Here's the drawing with two shaded views (mm, measured from the low corner). I have some questions. A direction names the side the tool comes from. Coordinates: 2 decimals unless noted, no trailing zeros. Loops run counter-clockwise (first coordinate to the right, second up) from the corner with the lowest first, then second, coordinate; pieces in that order, holes last.
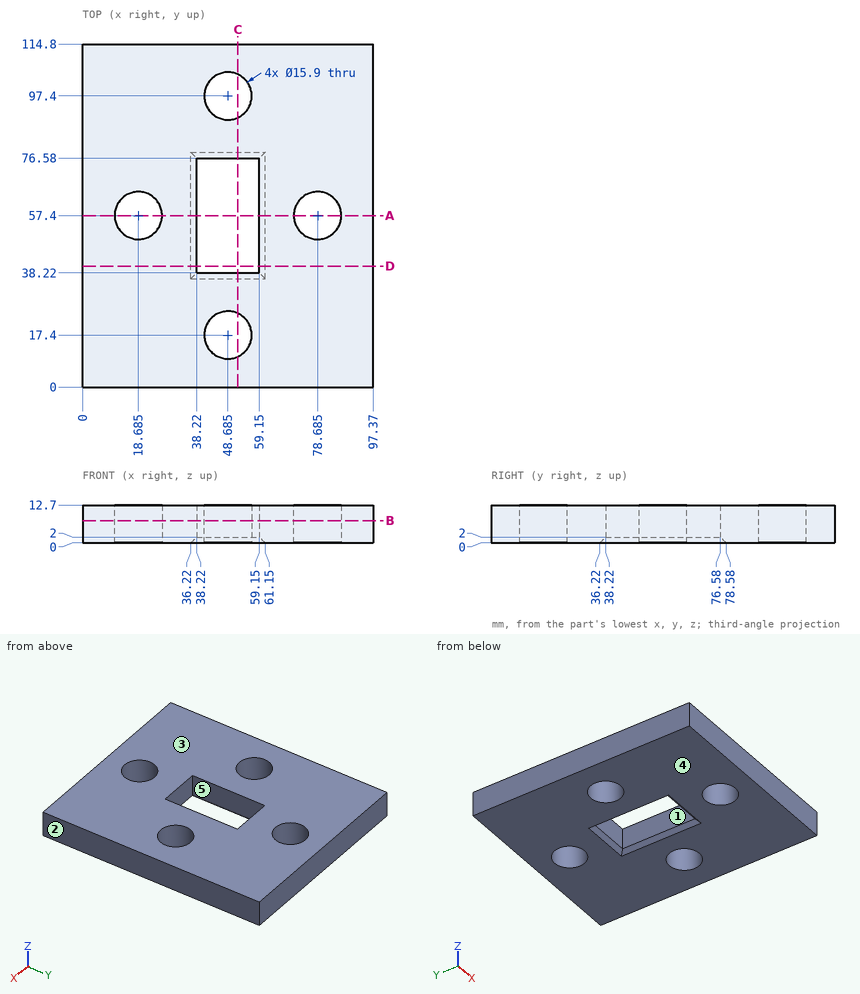
(1) I want a section at B-B on z = 7.5. Write out the boundary of the cut face in (x, y) (3 decimals), then the cut area to 3 significant figures.
Check values:
outline: (0, 0) - (97.37, 0) - (97.37, 114.8) - (0, 114.8) - close; hole circle Ø15.9 at (18.685, 57.4); hole (38.22, 38.22) - (59.15, 38.22) - (59.15, 76.58) - (38.22, 76.58) - close; hole circle Ø15.9 at (48.685, 17.4); hole circle Ø15.9 at (48.685, 97.4); hole circle Ø15.9 at (78.685, 57.4)
area: 9,580 mm2
(2) I want a section at A-A on y = 57.4. Write out the boundary of the cut face in (x, z) (3 decimals).
Check values:
outline: (0, 0) - (10.735, 0) - (10.735, 12.7) - (0, 12.7) - close; (26.635, 0) - (36.22, 0) - (38.22, 2) - (38.22, 12.7) - (26.635, 12.7) - close; (59.15, 2) - (61.15, 0) - (70.735, 0) - (70.735, 12.7) - (59.15, 12.7) - close; (86.635, 0) - (97.37, 0) - (97.37, 12.7) - (86.635, 12.7) - close
(3) I want a section at D-D on y = 40.5. Write out the boundary of the cut face in (x, z), then the cut area to 3 significant figures.
Check values:
outline: (0, 0) - (36.22, 0) - (38.22, 2) - (38.22, 12.7) - (0, 12.7) - close; (59.15, 2) - (61.15, 0) - (97.37, 0) - (97.37, 12.7) - (59.15, 12.7) - close
area: 967 mm2
(4) I want a section at C-C on x = 52. Write out the boundary of the cut face in (y, z).
Check values:
outline: (0, 0) - (10.17, 0) - (10.17, 12.7) - (0, 12.7) - close; (24.63, 0) - (36.22, 0) - (38.22, 2) - (38.22, 12.7) - (24.63, 12.7) - close; (76.58, 2) - (78.58, 0) - (90.17, 0) - (90.17, 12.7) - (76.58, 12.7) - close; (104.63, 0) - (114.8, 0) - (114.8, 12.7) - (104.63, 12.7) - close
(5) I'm going to push a flat-ended pin straight in: pin 1 (9.5 mm diameter, centred on x = 48.685, y = 97.4, fed in from -Z). Where does the tip first touch, or does it pass through?
Check values:
pin 1: passes through
(6) If we mould it in two halves opening along X, with no side actions, what happens to the marked faces 1, 2 and 3? For each: released by +X, released by -X, zero draft, split by the parting line, or undercut.
Check values:
face 1: undercut
face 2: released by +X
face 3: zero draft
(7) Which directions (+Z, -Z, +X, -X, +Y, -Y) give clear straight access to the entire face, cutting with the end or side of a thin tool? Please do the marked faces 4 and 5.
Check values:
face 4: -Z, +X, -X, +Y, -Y
face 5: +Z, -Z
(8) If I drill on probe 1 along Y at (x, z) = (43, 5.25); probe 2 along Y at (x, z) = (40, 4.5); probe 3 along Y at (x, z) = (52, 6.25), over which ranges is the centre line in solid material (lowest first)?
Check values:
probe 1: y = 0 to 11.84, 22.96 to 38.22, 76.58 to 91.84, 102.96 to 114.8
probe 2: y = 0 to 38.22, 76.58 to 114.8
probe 3: y = 0 to 10.17, 24.63 to 38.22, 76.58 to 90.17, 104.63 to 114.8
